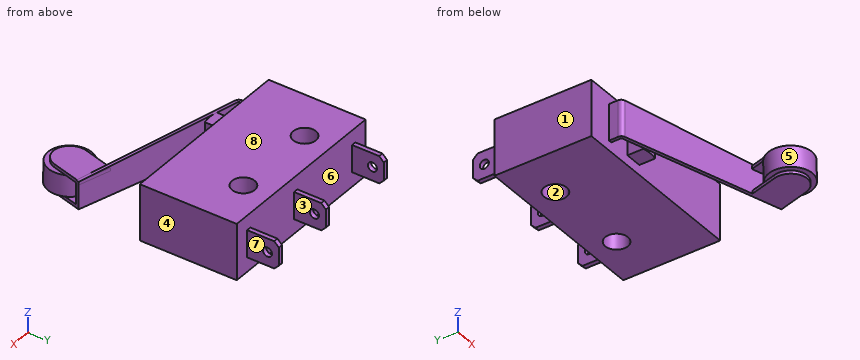
from build123d import *

# Parameters (mm, degrees)
SKETCH1_W           = 20
SKETCH1_H           = 10.7
BOSS_EXTRUDE1_DEPTH = 3.1
SKETCH2_W           = 0.5
SKETCH2_H           = 3.5
BOSS_EXTRUDE2_DEPTH = 1.5
CHAMFER1_SIZE       = 0.5
CUT_EXTRUDE1_REACH  = 25.448
SKETCH3_R           = 0.5
SKETCH4_R           = 1.25
CUT_EXTRUDE2_DEPTH  = 26.299802371
BOSS_EXTRUDE3_DEPTH = 2
DRAFT10_ANGLE       = 1.5
BOSS_EXTRUDE4_DEPTH = 0.35
SKETCH8_R           = 2.4
BOSS_EXTRUDE5_DEPTH = 2.330082213


with BuildPart() as part:
    # Sketch1 → Boss-Extrude1 (new, symmetric)
    with BuildSketch(Plane.XY):
        with Locations((10, 5.35)):
            Rectangle(SKETCH1_W, SKETCH1_H)
    extrude(amount=BOSS_EXTRUDE1_DEPTH, both=True)

    # Sketch2 → Boss-Extrude2 (add, symmetric)
    with BuildSketch(Plane.XY):
        with Locations((1.85, 12.45)):
            Rectangle(SKETCH2_W, SKETCH2_H)
        with Locations((18.15, 12.45)):
            Rectangle(SKETCH2_W, SKETCH2_H)
        with Locations((10.85, 12.45)):
            Rectangle(SKETCH2_W, SKETCH2_H)
    extrude(amount=BOSS_EXTRUDE2_DEPTH, both=True)

    # Chamfer1
    chamfer1_edges = [part.edges().sort_by_distance(p)[0] for p in [
        (1.85, 14.2, -1.5),
        (1.85, 14.2, 1.5),
        (18.15, 14.2, -1.5),
        (18.15, 14.2, 1.5),
        (10.85, 14.2, -1.5),
        (10.85, 14.2, 1.5),
    ]]
    chamfer(chamfer1_edges, length=CHAMFER1_SIZE)

    # Cut-Extrude1: up to this face of the body (flat: up to its plane)
    cut_extrude1_end = Plane(part.part.faces().sort_by_distance((1.6, 12.411382114, 0))[0])
    # Sketch3 → Cut-Extrude1 (cut, up to the picked face)
    with BuildSketch(Plane(origin=(18.4, 0, 0), x_dir=(0, 0, -1), z_dir=(1, 0, 0)), mode=Mode.PRIVATE) as cut_extrude1_sk1:
        with Locations(Location((0, 12.95, 0), (0, 0, 90))):
            Circle(SKETCH3_R)
    cut_extrude1_tool1 = split(extrude(cut_extrude1_sk1.sketch, amount=-CUT_EXTRUDE1_REACH, mode=Mode.PRIVATE), bisect_by=cut_extrude1_end, keep=Keep.BOTH, mode=Mode.PRIVATE)
    add(cut_extrude1_tool1.solids().sort_by(Axis((18.4, 12.95, 0), (-1, 0, 0)))[0], mode=Mode.SUBTRACT)

    # Sketch4 → Cut-Extrude2 (cut, through all)
    with BuildSketch(Plane(origin=(0, 0, -3.1), x_dir=(-1, 0, 0), z_dir=(0, 0, -1))):
        with Locations((-5.25, 7.7)):
            Circle(SKETCH4_R)
        with Locations((-14.75, 7.7)):
            Circle(SKETCH4_R)
    extrude(amount=-CUT_EXTRUDE2_DEPTH, mode=Mode.SUBTRACT)

    # Sketch5 → Boss-Extrude3 (add, symmetric)
    with BuildSketch(Plane.XY):
        with BuildLine():
            Line((2.75, 0), (2.75, -1))
            ThreePointArc((2.75, -1), (2.852752222, -1.303634983), (3.11877681, -1.482473289))
            Line((3.11877681, -1.482473289), (20.970288501, -6.337731302))
            Line((20.970288501, -6.337731302), (21.062144733, -6))
            Line((21.062144733, -6), (3.210633043, -1.144741987))
            ThreePointArc((3.210633043, -1.144741987), (3.130825667, -1.091090495), (3.1, -1))
            Line((3.1, -1), (3.1, 0))
            Line((3.1, 0), (2.75, 0))
        make_face()
        with BuildLine():
            Line((5.6, 0), (7.45, 0))
            Line((7.45, 0), (7.45, -1.75))
            ThreePointArc((7.45, -1.75), (6.525, -1.858422556), (5.6, -1.75))
            Line((5.6, -1.75), (5.6, 0))
        make_face()
    extrude(amount=BOSS_EXTRUDE3_DEPTH, both=True)

    # Draft10
    draft10_faces = [part.faces().sort_by_distance(p)[0] for p in [
        (11.436613636, -3.524482983, -2),
        (11.436613636, -3.524482983, 2),
    ]]
    draft(draft10_faces, Plane(origin=(3.279392904, -0.891929992, 0), x_dir=(0.26244637909853513, 0.9649465778467056, 0), z_dir=(0.9649465778467056, -0.26244637909853513, 0)), DRAFT10_ANGLE)

    # Sketch7 → Boss-Extrude4 (add)
    with BuildSketch(Plane(origin=(0.052748549, -0.014346562, -2.087562004), x_dir=(-0.9996809315410219, -0.0001699850736862716, -0.02525878497374093), z_dir=(0.02525935668815235, -0.006870045299250848, -0.9996573249755574))):
        with BuildLine():
            Line((-17.494148049, -5.03114496), (-21.016123341, -5.989367295))
            Line((-21.016123341, -5.989367295), (-20.097280006, -9.366603877))
            ThreePointArc((-20.097280006, -9.366603877), (-17.857181192, -10.648480355), (-16.575304714, -8.408381541))
            Line((-16.575304714, -8.408381541), (-17.494148049, -5.03114496))
        make_face()
    boss_extrude4 = extrude(amount=-BOSS_EXTRUDE4_DEPTH)

    # Mirror1: Boss-Extrude4 across plane
    add(boss_extrude4.mirror(Plane(origin=(0.014479585, -0.003938161, -0.573040064), x_dir=(0.9996809315475117, 0.00017358831123137617, 0.02525876021101414), z_dir=(0.02525935668815235, -0.006870045299250846, -0.9996573249755574))))

    # Sketch8 → Boss-Extrude5 (add)
    with BuildSketch(Plane(origin=(-0.014948604, 0.004065724, 0.591601811), x_dir=(-0.9996809315475117, -0.00017358831123137592, -0.025258760211014114), z_dir=(0.02525935668815233, -0.00687004529925084, -0.9996573249755573))):
        with Locations(Location((-18.336260335, -8.88755878, 0), (0, 0, 154.72118915))):
            Circle(SKETCH8_R)
    extrude(amount=BOSS_EXTRUDE5_DEPTH)


solid = part.part
Source: CAD feature listing. Evaluate the final solid. Frame: model axes, mm. Face numbers are marked on the shaded views. A direction names the side the tool comes from. Give positions to 0.01 mm unless a question says otherwise; leave off trailing zeros. Write each loop counter-clockwise with the first axis right and the second up, starting at its lowest first coordinate (ties: lowest second). Pieces come first, ordered by that corner, then holes. Notation, with made-up numbers: M 88,-14 L 119,-14 A23 ccw 119,12 Z; hole C -33,-11 d11. An arc over 180 degrees is marked long. Return JSON: item names as keys, results as strings. Group by question number.
1) Cut plane B-B, the plane x = 15. Output: boundary loops of the cut face in (y, z).
2) Set-up query: the marked faces 1, 2, 3, 4 and 5. Return all of +Z, -Z, +X, -X, +Y, -Y with unobstructed straight access to the full face (end or side cutting, diameter ignored); none if empty.
3) Pin query (flat end, axial travel): P1, Ø2, axis at x = 5.25, y = 7.7, coming from the -Z side; P2, Ø2, axis at y = 3, z = -1, coming from the +X side; P3, Ø5, axis at x = 10, y = -3.5, coming from the +Z side; P4, Ø0.5, axis at y = -0.5, z = 1, coming from the -X side. Return the tip coordinate at first contact, or that it passes through.
4) Pull-direction query (X, two-part tool) for the marked faces 6, 7 and 8; classes: pulls with the +X half, pulls with the -X half, needs draft (parallel to the pull), parting line crosses it, or undercut.
5) Material intervals for line 1 along Z through (x, y) = (10.95, 12.95); line 2 along Y through (x, z) = (18, 0.25); line 3 along Y through (x, z) = (5.25, 0), sorted ascending. Write a range as [from, to].
6) Cut plane D-D, the plane x = 12.25. Output: boundary loops of the cut face in (y, z).
7) Cut plane A-A, the plane y = 7.7. Output: boundary loops of the cut face in (x, z), plus the area to 3 significant figures.
8) Cut plane C-C, the plane y = 12.95. Output: boundary loops of the cut face in (x, z).
Recorded:
{
 "1": {"outline": "M -4.71,-1.68 L -4.35,-1.68 L -4.35,1.68 L -4.71,1.68 Z; M 0,-3.1 L 6.48,-3.1 L 6.48,3.1 L 0,3.1 Z; M 8.92,-3.1 L 10.7,-3.1 L 10.7,3.1 L 8.92,3.1 Z"},
 "2": {"face 1": "+Z, -Z, -X, +Y, -Y", "face 2": "+Z, -Z", "face 3": "+Z, -Z, +Y", "face 4": "+Z, -Z, +X, +Y", "face 5": "none"},
 "3": {"P1": "passes through", "P2": "stops at x = 20", "P3": "stops at z = 1.88", "P4": "stops at x = 2.75"},
 "4": {"face 6": "undercut", "face 7": "pulls with the +X half", "face 8": "needs draft"},
 "5": {"line 1": "z = [-1.5, -0.5], [0.5, 1.5]", "line 2": "y = [-11.26, -6.51], [-5.53, -5.17], [0, 12.52], [13.38, 14.2]", "line 3": "y = [-2.06, -1.7], [0, 6.45], [8.95, 10.7]"},
 "6": {"outline": "M -3.97,-1.75 L -3.6,-1.75 L -3.6,1.75 L -3.97,1.75 Z; M 0,-3.1 L 10.7,-3.1 L 10.7,3.1 L 0,3.1 Z"},
 "7": {"outline": "M 0,-3.1 L 4,-3.1 L 4,3.1 L 0,3.1 Z; M 6.5,-3.1 L 13.5,-3.1 L 13.5,3.1 L 6.5,3.1 Z; M 16,-3.1 L 20,-3.1 L 20,3.1 L 16,3.1 Z", "area": "93.0 mm²"},
 "8": {"outline": "M 1.6,-1.5 L 2.1,-1.5 L 2.1,-0.5 L 1.6,-0.5 Z; M 1.6,0.5 L 2.1,0.5 L 2.1,1.5 L 1.6,1.5 Z; M 10.6,-1.5 L 11.1,-1.5 L 11.1,-0.5 L 10.6,-0.5 Z; M 10.6,0.5 L 11.1,0.5 L 11.1,1.5 L 10.6,1.5 Z; M 17.9,-1.5 L 18.4,-1.5 L 18.4,-0.5 L 17.9,-0.5 Z; M 17.9,0.5 L 18.4,0.5 L 18.4,1.5 L 17.9,1.5 Z"}
}
